from build123d import *

# Parameters (mm, degrees)
SKETCH1_R               = 4.765
BOSS_EXTRUDE1_DEPTH     = 9.5
CHAMFER1_SIZE           = 7.62
CHAMFER1_SIZE2          = 2.54
CHAMFER2_SIZE           = 2.54
CHAMFER2_SIZE2          = 7.62
CHAMFER2_PART_2_SIZE    = 2.54
CHAMFER2_PART_2_SIZE2   = 7.62
SKETCH5_W               = 9.53
SKETCH5_H               = 9.53
CUT_EXTRUDE1_DEPTH      = 20.54
CUT_EXTRUDE2_DEPTH      = 10.77
CUT_EXTRUDE2_DEPTH_BACK = 10.77
SKETCH7_R               = 1.59
CUT_EXTRUDE3_DEPTH      = 10.5000001
CUT_EXTRUDE3_DEPTH_BACK = 10.5000001


with BuildPart() as part:
    # Sketch1 → Boss-Extrude1 (new body, symmetric)
    with BuildSketch(Plane.XY):
        with BuildLine():
            Line((0, 9.77), (-22.23, 9.77))
            Line((-22.23, 9.77), (-22.23, 4.77))
            Line((-22.23, 4.77), (-9.711509246, -1.067468107))
            ThreePointArc((-9.711509246, -1.067468107), (-5.877874817, -7.804068659), (1.655323868, -9.628748771))
            Line((1.655323868, -9.628748771), (28.58, -5))
            Line((28.58, -5), (28.58, 0))
            Line((28.58, 0), (9.77, 0))
            ThreePointArc((9.77, 0), (6.908433252, 6.908433252), (0, 9.77))
        make_face()
        Circle(SKETCH1_R, mode=Mode.SUBTRACT)
    extrude(amount=BOSS_EXTRUDE1_DEPTH, both=True)

    # Chamfer1
    chamfer1_edges = [part.edges().sort_by_distance(p)[0] for p in [
        (-22.23, 7.27, -9.5),
        (28.58, -2.5, -9.5),
    ]]
    chamfer1_side = [part.faces().sort_by_distance(p)[0] for p in [
        (-11.115, 9.225622585, -9.5),
    ]]
    chamfer(chamfer1_edges, length=CHAMFER1_SIZE, length2=CHAMFER1_SIZE2, reference=chamfer1_side[0])

    # Chamfer2
    chamfer2_edges = [part.edges().sort_by_distance(p)[0] for p in [
        (-22.23, 7.27, 9.5),
    ]]
    chamfer2_side = [part.faces().sort_by_distance(p)[0] for p in [
        (-22.23, 7.27, 1.27),
    ]]
    chamfer(chamfer2_edges, length=CHAMFER2_SIZE, length2=CHAMFER2_SIZE2, reference=chamfer2_side[0])

    # Chamfer2 part 2
    chamfer2_part_2_edges = [part.edges().sort_by_distance(p)[0] for p in [
        (28.58, -2.5, 9.5),
    ]]
    chamfer2_part_2_side = [part.faces().sort_by_distance(p)[0] for p in [
        (28.58, -2.5, 1.27),
    ]]
    chamfer(chamfer2_part_2_edges, length=CHAMFER2_PART_2_SIZE, length2=CHAMFER2_PART_2_SIZE2, reference=chamfer2_part_2_side[0])

    # Sketch5 → Cut-Extrude1 (cut, through all)
    with BuildSketch(Plane(origin=(0, 9.77, 0), x_dir=(1, 0, 0), z_dir=(0, 1, 0))):
        with Locations((-17.465, 0)):
            Rectangle(SKETCH5_W, SKETCH5_H)
        with Locations((23.815, 0)):
            Rectangle(SKETCH5_W, SKETCH5_H)
    extrude(amount=-CUT_EXTRUDE1_DEPTH, mode=Mode.SUBTRACT)

    # Sketch6 → Cut-Extrude2 (cut, two sides)
    with BuildSketch(Plane(origin=(0, 0, 0), x_dir=(1, 0, 0), z_dir=(0, 1, 0))) as cut_extrude2_sk:
        with BuildLine():
            Line((-3.81, 5.08), (6.35, 5.08))
            ThreePointArc((6.35, 5.08), (11.43, 0), (6.35, -5.08))
            Line((6.35, -5.08), (-3.81, -5.08))
            ThreePointArc((-3.81, -5.08), (-8.89, 0), (-3.81, 5.08))
        make_face()
    extrude(amount=CUT_EXTRUDE2_DEPTH, mode=Mode.SUBTRACT)
    extrude(cut_extrude2_sk.sketch, amount=-CUT_EXTRUDE2_DEPTH_BACK, mode=Mode.SUBTRACT)

    # Sketch7 → Cut-Extrude3 (cut, two sides)
    with BuildSketch(Plane.XY) as cut_extrude3_sk:
        with Locations((-19.69, 7.23)):
            Circle(SKETCH7_R)
        with Locations((26.04, -2.54)):
            Circle(SKETCH7_R)
    extrude(amount=CUT_EXTRUDE3_DEPTH, mode=Mode.SUBTRACT)
    extrude(cut_extrude3_sk.sketch, amount=-CUT_EXTRUDE3_DEPTH_BACK, mode=Mode.SUBTRACT)


solid = part.part
CAD build for the part. Positions are in the model's coordinates, mm. A direction names the side the tool comes from. Round coordinates to 2 decimals unless told otherwise and drop trailing zeros. Loops run counter-clockwise (first coordinate to the right, second up) from the corner with the lowest first, then second, coordinate; pieces in that order, holes last.
(1) Cut at B-B (z = -2.5). Give the cut face in (x, y), plus the area to 3 significant figures.
(2) Wall check: line 1 along Z through (x, y) = (6, -5); line 2 along X through (y, z) = (-2.54, -6.7); line 3 along X through (y, z) = (7.23, 6.9). Give the ranges that are in metal, low to high.
(3) Cut at A-A (y = 4). Give the cut face in (x, z) (3 decimals), plus the area to 3 significant figures.
(4) Which spindle directions (+Z, -Z, +X, -X, +Y, -Y) get a long thin tool onto all of the face, cutting with end or side? Do faces 4 (the flat face through (-22.23, 7, 6)), 5 (the cylindrical face through (-8.89, 2.34, 0.11)), 6 (the flat face through (-12.7, 5, 0)), 7 (the flat face through (23.977, -3.199, -8.494)), 8 (the flat face through (23, -3, -4.765)). Say none if no direction does.
(5) Drop flat-ended pins along their axis: pin 1 (2 mm diameter, centred on y = -2, z = -2, fed in from +X); pin 2 (4 mm diameter, centred on x = 26.04, y = -2.54, fed in from +Z); pin 3 (7.5 mm diameter, centred on x = 26, y = -2, fed in from -Z). Give the stop position or say it passes through.
(6) Two-plate mould, pull along X, no slides. Class faces 1 (the flat face through (-12, 0, 0)), 2 (the cylindrical face through (-18.173, 7.708, 6.129)), 3 (the flat face through (-16, 6, -4.765)): +X half, -X half, draft (parallel to the pull), parting line (faces both ways), or undercut.
(7) Cut at D-D (x = 26.04). Give the cut face in (y, z) (3 decimals), plus the area to 3 significant figures.
(8) Cut at C-C (x = 10.5). Give the cut face in (y, z), plus the area to 3 significant figures.
Findings below:
1. outline: (-12.7, 0.33) - (-9.71, -1.07) arc R9.77 ccw to (-8.23, -5.26) - (-8.23, 9.77) - (-12.7, 9.77) - close; (10.77, -8.06) - (19.05, -6.64) - (19.05, 0) - (10.77, 0) - close
1. area: 111 mm2
2. line 1: z = -9.5 to -5.08, 5.08 to 9.5
2. line 2: x = -9.43 to -4.03, 4.03 to 24.45, 27.63 to 28.58
2. line 3: x = -22.23 to -21.28, -18.1 to 6.57
3. outline: (-20.579, -7.51) - (-14.61, -9.5) - (-2.589, -9.5) - (-2.589, -5.08) - (-3.81, -5.08) arc R5.08 cw to (-3.81, 5.08) - (-2.589, 5.08) - (-2.589, 9.5) - (-14.61, 9.5) - (-20.579, 7.51) - (-20.579, 4.765) - (-12.7, 4.765) - (-12.7, -4.765) - (-20.579, -4.765) - close; (2.589, -9.5) - (8.914, -9.5) - (8.914, -4.386) arc R5.08 cw to (6.35, -5.08) - (2.589, -5.08) - close; (2.589, 5.08) - (6.35, 5.08) arc R5.08 cw to (8.914, 4.386) - (8.914, 9.5) - (2.589, 9.5) - close
3. area: 259 mm2
4. face 4: +Z, -Z, -X, +Y, -Y
4. face 5: +Y, -Y
4. face 6: -X, +Y, -Y
4. face 7: -Z, +X, +Y, -Y
4. face 8: +X, +Y, -Y
5. pin 1: stops at x = 19.05
5. pin 2: stops at z = 8.47
5. pin 3: stops at z = -9.07
6. face 1: -X half
6. face 2: undercut
6. face 3: draft
7. outline: (-5.437, -7.807) - (-4.13, -7.807) - (-4.13, -4.765) - (-5.437, -4.765) - close; (-5.437, 4.765) - (-4.13, 4.765) - (-4.13, 7.807) - (-5.437, 7.807) - close; (-0.95, -7.807) - (0, -7.807) - (0, -4.765) - (-0.95, -4.765) - close; (-0.95, 4.765) - (0, 4.765) - (0, 7.807) - (-0.95, 7.807) - close
7. area: 13.7 mm2
8. outline: (-8.11, -9.5) - (0, -9.5) - (0, -2.93) - (-8.11, -2.93) - close; (-8.11, 2.93) - (0, 2.93) - (0, 9.5) - (-8.11, 9.5) - close
8. area: 107 mm2
